Verification items for the finished model (mm, model axes). Face numbers are marked on the shaded views. Round coordinates to 2 decimals unless told otherwise and drop trailing zeros. Loops run counter-clockwise (first coordinate to the right, second up) from the corner with the lowest first, then second, coordinate; pieces in that order, holes last. Notation, with made-up numbers: M 61,89 L 111,89 A8 ccw 111,100 Z; hole C 27,-19.5 d8. An arc over 180 degrees is marked long. Answer as CSV lines item,"result".
Autodesk Inventor part; units mm, degrees
ref_plane "YZ Plane" through (0, 0, 0) normal (1, 0, 0) x (0, 1, 0)
ref_plane "XZ Plane" through (0, 0, 0) normal (0, 1, 0) x (-1, 0, 0)
ref_plane "XY Plane" through (0, 0, 0) normal (0, 0, 1) x (1, 0, 0)
sketch "Sketch1" plane through (0, 0, 0) normal (0, 1, 0) x (-1, 0, 0)
  circle A0 centre (0, 0) radius 9.525
  circle A1 centre (0, 0) radius 3
  circle A2 centre (4.7625, 4.7625) radius 1.5875
  circle A3 centre (-4.7625, 4.7625) radius 1.5875
  circle A4 centre (-4.7625, -4.7625) radius 1.5875
  circle A5 centre (4.7625, -4.7625) radius 1.5875
  dimension "d0" = 19.05
  dimension "d1" = 3.175
  dimension "d4" = 360
  dimension "d6" = 6
extrude "Extrusion1" add sketch "Sketch1" along normal blind 3.175
properties part number "Flip up and down (motor to shaft ring)"
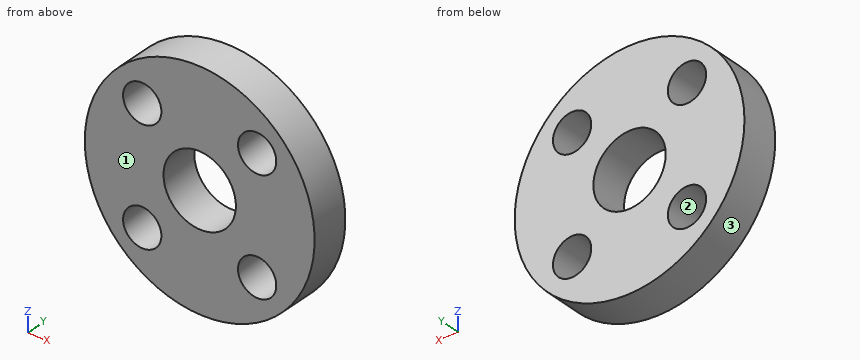
1) Material ranges on probe 1 along Z at (x, y) = (-4.75, 0.25); probe 2 along Z at (x, y) = (-5.5, 1.45); probe 3 along Z at (x, y) = (0, 1.75) (3 decimals), recorded low to high.
Here are the results:
probe 1,"z = -8.26 to -6.35, -3.18 to 3.18, 6.35 to 8.26"
probe 2,"z = -7.78 to -6.17, -3.36 to 3.36, 6.17 to 7.78"
probe 3,"z = -9.525 to -3, 3 to 9.525"
2) Section check B-B (x = 0). Record the cut outline in (y, z) (3 decimals), plus the area to 3 significant figures.
Here are the results:
outline,"M 0,-9.525 L 3.175,-9.525 L 3.175,-3 L 0,-3 Z; M 0,3 L 3.175,3 L 3.175,9.525 L 0,9.525 Z"
area,"41.4 mm^2"
3) Draft check along Z on the marked faces 1, 2 and 3. Enter one of: +Z half, -Z half, draft (parallel to the pull), parting line (faces both ways), or undercut.
Here are the results:
face 1,"draft"
face 2,"undercut"
face 3,"parting line"
4) Section check C-C (y = 2.9). State how many separate pieces and enclosed holes the cut face has, plus the area to 3 significant figures.
Here are the results:
separate pieces,"1"
enclosed holes,"5"
area,"225 mm^2"
5) Section check A-A (z = 0). Record the cut outline in (x, y) (3 decimals).
Here are the results:
outline,"M -9.525,0 L -3,0 L -3,3.175 L -9.525,3.175 Z; M 3,0 L 9.525,0 L 9.525,3.175 L 3,3.175 Z"
6) Section check D-D (z = 3.75). Record the cut outline in (x, y) (3 decimals), plus the area to 3 significant figures.
Here are the results:
outline,"M -8.756,0 L -5.985,0 L -5.985,3.175 L -8.756,3.175 Z; M -3.54,0 L 3.54,0 L 3.54,3.175 L -3.54,3.175 Z; M 5.985,0 L 8.756,0 L 8.756,3.175 L 5.985,3.175 Z"
area,"40.1 mm^2"
7) Go/stop test with flat-tipped pins: pin 1 (1.9 mm diameter, centred on x = -4.76, z = 4.76, fed in from +Y); pin 2 (1 mm diameter, centred on y = 2.5, z = 6, fed in from +X). Record where each tip stops, or that it passes through.
Here are the results:
pin 1,"passes through"
pin 2,"stops at x = 7.78"
